Can you work these out from the model? Positions are in its coordinate system, mm. Face numbers are marked on the shaded views. A direction names the side the tool comes from. Give positions to 0.01 mm unless a question says otherwise; leave off trailing zeros. Order: outer loops, then holes, each group sorted by start corner. A loop starts at its lowest first (then second) coordinate and runs counter-clockwise, first axis right, second up. Notation, with made-up numbers: (32.25, 11) - (67.25, 11) arc R23 cw to (67.25, 26) - close; hole circle Ø10 at (38, 17). An arc over 180 degrees is marked (long way). Answer as a JSON object with one key per item and string values.
```python
from build123d import *

# Parameters (mm, degrees)
SKETCH1_R           = 19.5
BOSS_EXTRUDE1_DEPTH = 15
SKETCH2_R           = 21
BOSS_EXTRUDE2_DEPTH = 2
SKETCH3_R           = 50
BOSS_EXTRUDE3_DEPTH = 5
CUT_EXTRUDE2_DEPTH  = 5
CUT_EXTRUDE3_DEPTH  = 2.5
SKETCH8_R           = 2.5
CUT_EXTRUDE4_DEPTH  = 20.5
BOSS_EXTRUDE4_DEPTH = 5
FILLET1_R           = 1
SKETCH10_R          = 50
SKETCH10_R_2        = 21
CUT_EXTRUDE5_DEPTH  = 28


with BuildPart() as part:
    # Sketch1 → Boss-Extrude1 (new body)
    with BuildSketch(Plane.XY):
        Circle(SKETCH1_R)
    extrude(amount=BOSS_EXTRUDE1_DEPTH)

    # Sketch2 → Boss-Extrude2 (add)
    with BuildSketch(Plane.XY.offset(15)):
        Circle(SKETCH2_R)
    extrude(amount=BOSS_EXTRUDE2_DEPTH)

    # Sketch3 → Boss-Extrude3 (add)
    with BuildSketch(Plane.XY.offset(17)):
        Circle(SKETCH3_R)
    extrude(amount=BOSS_EXTRUDE3_DEPTH)

    # Sketch4 → Cut-Extrude2 (cut)
    with BuildSketch(Plane(origin=(0, 0, 17), x_dir=(-1, 0, 0), z_dir=(0, 0, -1))):
        with BuildLine():
            ThreePointArc((-18.186533, -10.5), (-21, 0), (-18.186533, 10.5))
            Line((-18.186533, 10.5), (-36.669606, 21.484645))
            ThreePointArc((-36.669606, 21.484645), (-42.499783, 0.135723), (-36.80608, -21.25))
            Line((-36.80608, -21.25), (-18.186533, -10.5))
        make_face()
        with BuildLine():
            Line((-21.25, 36.80608), (-10.5, 18.186533))
            ThreePointArc((-10.5, 18.186533), (0, 21), (10.5, 18.186533))
            Line((10.5, 18.186533), (21.484645, 36.669606))
            ThreePointArc((21.484645, 36.669606), (0.135723, 42.499783), (-21.25, 36.80608))
        make_face()
        with BuildLine():
            Line((36.80608, 21.25), (18.186533, 10.5))
            ThreePointArc((18.186533, 10.5), (20.284442, 5.4352), (21, 0))
            ThreePointArc((21, 0), (20.284442, -5.4352), (18.186533, -10.5))
            Line((18.186533, -10.5), (36.669606, -21.484645))
            ThreePointArc((36.669606, -21.484645), (42.499783, -0.135723), (36.80608, 21.25))
        make_face()
    extrude(amount=-CUT_EXTRUDE2_DEPTH, mode=Mode.SUBTRACT)

    # Sketch5 → Cut-Extrude3 (cut)
    with BuildSketch(Plane.XY.offset(22)):
        with BuildLine():
            Line((-15, -47.69696), (-15, -27.69696))
            Line((-15, -27.69696), (15, -27.69696))
            Line((15, -27.69696), (15, -47.69696))
            ThreePointArc((15, -47.69696), (0, -50), (-15, -47.69696))
        make_face()
    extrude(amount=-CUT_EXTRUDE3_DEPTH, mode=Mode.SUBTRACT)

    # Sketch8 → Cut-Extrude4 (cut, through all)
    with BuildSketch(Plane.XY.offset(19.5)):
        with Locations((-7.5, -37.69696)):
            Circle(SKETCH8_R)
        with Locations((7.5, -37.69696)):
            Circle(SKETCH8_R)
    extrude(amount=-CUT_EXTRUDE4_DEPTH, mode=Mode.SUBTRACT)

    # Sketch9 → Boss-Extrude4 (add)
    with BuildSketch(Plane.XY.offset(22)):
        with BuildLine():
            Line((-36.80608, 21.25), (-43.30127, 25))
            ThreePointArc((-43.30127, 25), (-49.999665, -0.183068), (-43.117043, -25.31641))
            Line((-43.117043, -25.31641), (-36.669606, -21.484645))
            ThreePointArc((-36.669606, -21.484645), (-42.499783, -0.135723), (-36.80608, 21.25))
        make_face()
        with BuildLine():
            Line((-21.484645, 36.669606), (-25.31641, 43.117043))
            ThreePointArc((-25.31641, 43.117043), (-0.183068, 49.999665), (25, 43.30127))
            Line((25, 43.30127), (21.25, 36.80608))
            ThreePointArc((21.25, 36.80608), (-0.135723, 42.499783), (-21.484645, 36.669606))
        make_face()
        with BuildLine():
            Line((36.669606, 21.484645), (43.117043, 25.31641))
            ThreePointArc((43.117043, 25.31641), (49.999665, 0.183068), (43.30127, -25))
            Line((43.30127, -25), (36.80608, -21.25))
            ThreePointArc((36.80608, -21.25), (42.499783, 0.135723), (36.669606, 21.484645))
        make_face()
    extrude(amount=BOSS_EXTRUDE4_DEPTH)

    # Fillet1
    fillet1_edges = [part.edges().sort_by_distance(p)[0] for p in [
        (-0.135723, 42.499783, 27),
        (23.125, 40.053675, 27),
        (-0.183068, 49.999665, 27),
        (-23.400528, 39.893324, 27),
        (42.499783, 0.135723, 27),
        (40.053675, -23.125, 27),
        (49.999665, 0.183068, 27),
        (39.893324, 23.400528, 27),
        (-42.499783, -0.135723, 27),
        (-40.053675, 23.125, 27),
        (-49.999665, -0.183068, 27),
        (-39.893324, -23.400528, 27),
    ]]
    fillet(fillet1_edges, radius=FILLET1_R)

    # Sketch10 → Cut-Extrude5 (cut, through all)
    with BuildSketch(Plane(origin=(0, 0, 0), x_dir=(-1, 0, 0), z_dir=(0, 0, -1))):
        Circle(SKETCH10_R)
        Circle(SKETCH10_R_2, mode=Mode.SUBTRACT)
    extrude(amount=-CUT_EXTRUDE5_DEPTH, mode=Mode.SUBTRACT)


solid = part.part
```
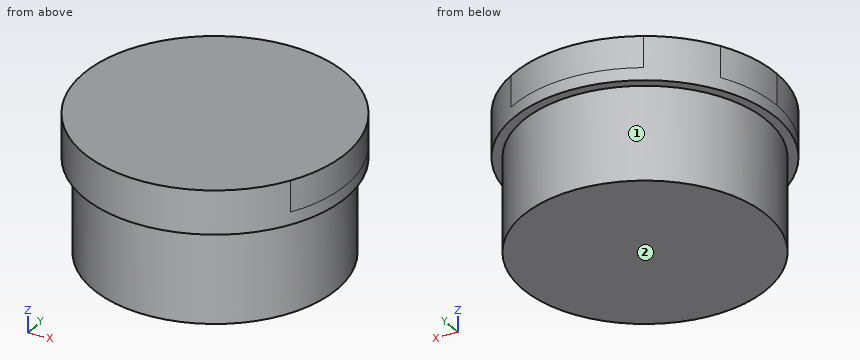
Q1. Which directions (+Z, -Z, +X, -X, +Y, -Y) give clear straight access to the entire face, cutting with the end or side of a thin tool? Please do the marked faces 1 and 2.
Recorded:
{"face 1": "-Z", "face 2": "-Z, +X, -X, +Y, -Y"}
Q2. If we section it at D-D, the plane y = 3: Please give me the cut outline in (x, z), then the cut area to 3 significant figures.
Recorded:
{"outline": "(-20.78, 15) - (-19.27, 15) - (-19.27, 0) - (19.27, 0) - (19.27, 15) - (20.78, 15) - (20.78, 22) - (-20.78, 22) - close", "area": "869 mm^2"}
Q3. I'm going to push flat-ended pins straight in: pin 1 Ø1.5 at (y, z) = (10, 5) entering from -X; pin 2 Ø3 at (y, z) = (-8, 10.5) entering from +X; pin 3 Ø10 at (x, z) = (-8.5, 19) entering from +Y. Where does each tip first touch, or does it pass through?
Recorded:
{"pin 1": "stops at x = -17.17", "pin 2": "stops at x = 18.38", "pin 3": "stops at y = 20.71"}
Q4. If we section it at B-B, the plane x = 0: Please give me the cut outline in (y, z).
Recorded:
{"outline": "(-21, 15) - (-19.5, 15) - (-19.5, 0) - (19.5, 0) - (19.5, 15) - (21, 15) - (21, 22) - (-21, 22) - close"}
Q5. I need wall thicknesses on L1, parallel to Z at x = -6, y = -19; L2, parallel to Y at x = -14, z = 14.75; L3, parallel to Y at x = 15, z = 14.5. Which ranges of each line are inside material? Lowest first, please.
Recorded:
{"L1": "z = 15 to 22", "L2": "y = -13.57 to 13.57", "L3": "y = -12.46 to 12.46"}
Q6. If we section it at A-A, the plane y = 16: Please give me the cut outline in (x, z).
Recorded:
{"outline": "(-13.6, 15) - (-11.15, 15) - (-11.15, 0) - (11.15, 0) - (11.15, 15) - (13.6, 15) - (13.6, 22) - (-13.6, 22) - close"}
Q7. If we section it at C-C, the plane z = 3: Please give me the cut outline in (x, y), then the cut area to 3 significant figures.
Recorded:
{"outline": "circle Ø39 at (0, 0)", "area": "1,190 mm^2"}
